Work out the finished part from the listing and answer in its coordinate system (mm). Round coordinates to 2 decimals unless told otherwise and drop trailing zeros. Order: outer loops, then holes, each group sorted by start corner. A loop starts at its lowest first (then second) coordinate and runs counter-clockwise, first axis right, second up. Notation, with made-up numbers: M 42.5,-2.75 L 62.5,-2.75 A18 cw 62.5,5.25 Z; hole C -4,-4.5 d7. An arc over 180 degrees is marked long. Return JSON: item names as keys, results as strings.
from build123d import *

# Parameters (mm, degrees)
SKETCH1_R           = 2
BOSS_EXTRUDE1_DEPTH = 20
SKETCH2_R           = 3.2
BOSS_EXTRUDE2_DEPTH = 1.7
BOSS_EXTRUDE2_TAPER = 32
SKETCH3_W           = 0.5
SKETCH3_H           = 2.258378485
SKETCH3_H_2         = 2.241621515
SKETCH3_W_2         = 2.234727157
SKETCH3_H_3         = 0.5
SKETCH3_W_3         = 2.265272843
CUT_EXTRUDE1_DEPTH  = 0.3


with BuildPart() as part:
    # Sketch1 → Boss-Extrude1 (new body)
    with BuildSketch(Plane(origin=(0, 0, 0), x_dir=(1, 0, 0), z_dir=(0, 1, 0))):
        Circle(SKETCH1_R)
    extrude(amount=BOSS_EXTRUDE1_DEPTH)

    # Sketch2 → Boss-Extrude2 (add)
    with BuildSketch(Plane(origin=(0, 20, 0), x_dir=(1, 0, 0), z_dir=(0, 1, 0))):
        Circle(SKETCH2_R)
    extrude(amount=-BOSS_EXTRUDE2_DEPTH, taper=BOSS_EXTRUDE2_TAPER)

    # Sketch3 → Cut-Extrude1 (cut)
    with BuildSketch(Plane(origin=(0, 20, 0), x_dir=(1, 0, 0), z_dir=(0, 1, 0))):
        with Locations((-0.015272843, 1.370810757)):
            Rectangle(SKETCH3_W, SKETCH3_H)
        with Locations((-0.015272843, -1.379189243)):
            Rectangle(SKETCH3_W, SKETCH3_H_2)
        with Locations((-1.382636421, -0.008378485)):
            Rectangle(SKETCH3_W_2, SKETCH3_H_3)
        with Locations((1.367363579, -0.008378485)):
            Rectangle(SKETCH3_W_3, SKETCH3_H_3)
        with Locations((-0.015272843, -0.008378485)):
            Rectangle(SKETCH3_W, SKETCH3_H_3)
    extrude(amount=-CUT_EXTRUDE1_DEPTH, mode=Mode.SUBTRACT)


solid = part.part
Item 1: Find section A-A (x = 0). Determine the outline of the cut face in (y, z).
Output:
{"outline": "M 0,-2 L 18.3,-2 L 18.3,-2.14 L 20,-3.2 L 20,-2.5 L 19.7,-2.5 L 19.7,2.5 L 20,2.5 L 20,3.2 L 18.3,2.14 L 18.3,2 L 0,2 Z"}
Item 2: Each of these flat-tipped pins is pushed along its axis until it touches: pin 1 (1 mm diameter, centred on y = 2.5, z = 0, fed in from +X); pin 2 (1 mm diameter, centred on x = -0.5, y = 10, fed in from -Z); pin 3 (1.5 mm diameter, centred on y = 12, z = -2.5, fed in from -X). Where does it stop, or does it pass through?
Output:
{"pin 1": "stops at x = 2", "pin 2": "stops at z = -2", "pin 3": "stops at x = -0.97"}
Item 3: Consider line 1 along Z through (x, y) = (0, 15); line 2 along Z through (x, y) = (-1, 11); line 3 along X through (y, z) = (5.5, -1.75). Determine where each line is inside the solid, lowest interval first. Write a range as [from, to].
Output:
{"line 1": "z = [-2, 2]", "line 2": "z = [-1.73, 1.73]", "line 3": "x = [-0.97, 0.97]"}
Item 4: Find section B-B (y = 8.25). Determine the outline of the cut face in (x, z), plus the area to 3 significant figures.
Output:
{"outline": "C 0,0 d4", "area": "12.6 mm^2"}
Item 5: The mould has two halves that part along X. Classify faces 1 (the flat face through (0, 19.7, 0)), 2 (the flat face through (0, 0, 0)), 3 (the cylindrical face through (0, 9, 2)): pulls with the +X half, pulls with the -X half, needs draft (parallel to the pull), parting line crosses it, or undercut.
Output:
{"face 1": "undercut", "face 2": "needs draft", "face 3": "parting line crosses it"}
